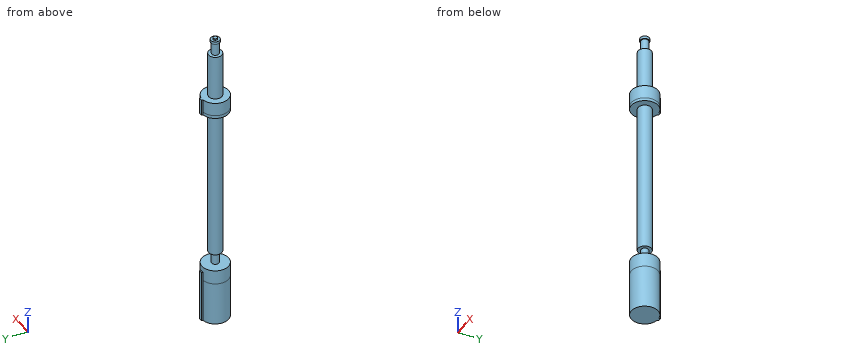
from build123d import *

# Parameters (mm, degrees)
CROQUIS1_R               = 4
SALIENTE_EXTRUIR1_DEPTH  = 135
CROQUIS2_R               = 5
SALIENTE_EXTRUIR2_DEPTH  = 3
SALIENTE_EXTRUIR3_DEPTH  = 1.8
CROQUIS4_R               = 7.5
SALIENTE_EXTRUIR4_DEPTH  = 120.9
CROQUIS5_R               = 15
SALIENTE_EXTRUIR5_DEPTH  = 15
CROQUIS7_W               = 4
CROQUIS7_H               = 3
SALIENTE_EXTRUIR6_DEPTH  = 15
SALIENTE_EXTRUIR7_DEPTH  = 3.4
CROQUIS9_R               = 15
SALIENTE_EXTRUIR8_DEPTH  = 6
CROQUIS10_R              = 15
SALIENTE_EXTRUIR9_DEPTH  = 10
SALIENTE_EXTRUIR10_DEPTH = 49


with BuildPart() as part:
    # Croquis1 → Saliente-Extruir1 (new, symmetric)
    with BuildSketch(Plane.XY):
        Circle(CROQUIS1_R)
    extrude(amount=SALIENTE_EXTRUIR1_DEPTH, both=True)

    # Croquis2 → Saliente-Extruir2 (add)
    with BuildSketch(Plane.XY.offset(135)):
        Circle(CROQUIS2_R)
    extrude(amount=SALIENTE_EXTRUIR2_DEPTH)

    # Croquis3 → Saliente-Extruir3 (add)
    with BuildSketch(Plane.XY.offset(138)):
        Polygon((0, 2.5), (-2.165063509, 1.25), (-2.165063509, -1.25), (0, -2.5), (2.165063509, -1.25), (2.165063509, 1.25), align=None)
    extrude(amount=SALIENTE_EXTRUIR3_DEPTH)

    # Croquis4 → Saliente-Extruir4 (add, symmetric)
    with BuildSketch(Plane.XY):
        Circle(CROQUIS4_R)
    extrude(amount=SALIENTE_EXTRUIR4_DEPTH, both=True)

    # Croquis5 → Saliente-Extruir5 (add)
    with BuildSketch(Plane(origin=(0, 0, 70), x_dir=(-1, 0, 0), z_dir=(0, 0, -1))):
        Circle(CROQUIS5_R)
    extrude(amount=SALIENTE_EXTRUIR5_DEPTH)

    # Croquis7 → Saliente-Extruir6 (add)
    with BuildSketch(Plane.XY.offset(70)):
        with Locations((0, 15)):
            Rectangle(CROQUIS7_W, CROQUIS7_H)
    extrude(amount=-SALIENTE_EXTRUIR6_DEPTH)

    # Croquis8 → Saliente-Extruir7 (add)
    with BuildSketch(Plane(origin=(0, 0, 55), x_dir=(-1, 0, 0), z_dir=(0, 0, -1))):
        with BuildLine():
            Line((2, 14.866068747), (2, 16.5))
            Line((2, 16.5), (-2, 16.5))
            Line((-2, 16.5), (-2, 14.866068747))
            ThreePointArc((-2, 14.866068747), (0, -15), (2, 14.866068747))
        make_face()
    extrude(amount=SALIENTE_EXTRUIR7_DEPTH)

    # Croquis9 → Saliente-Extruir8 (add)
    with BuildSketch(Plane(origin=(0, 0, -135), x_dir=(-1, 0, 0), z_dir=(0, 0, -1))):
        Circle(CROQUIS9_R)
    extrude(amount=SALIENTE_EXTRUIR8_DEPTH)

    # Croquis10 → Saliente-Extruir9 (add)
    with BuildSketch(Plane(origin=(0, 0, -141), x_dir=(-1, 0, 0), z_dir=(0, 0, -1))):
        with Locations(Location((0, 0, 0), (0, 0, 97.662255661))):
            Circle(CROQUIS10_R)
        with BuildLine():
            Line((-2, 16.5), (-2, 14.866068747))
            ThreePointArc((-2, 14.866068747), (0, 15), (2, 14.866068747))
            Line((2, 14.866068747), (2, 16.5))
            Line((2, 16.5), (-2, 16.5))
        make_face()
    extrude(amount=SALIENTE_EXTRUIR9_DEPTH)

    # Croquis11 → Saliente-Extruir10 (add)
    with BuildSketch(Plane(origin=(0, 0, -151), x_dir=(-1, 0, 0), z_dir=(0, 0, -1))):
        with BuildLine():
            Line((2, 14.866068747), (2, 16.5))
            Line((2, 16.5), (-2, 16.5))
            Line((-2, 16.5), (-2, 14.866068747))
            ThreePointArc((-2, 14.866068747), (0, -15), (2, 14.866068747))
        make_face()
    extrude(amount=SALIENTE_EXTRUIR10_DEPTH)


solid = part.part
The listing builds one solid part. Answer for the finished solid, in the listing's coordinates (mm). Round coordinates to 2 decimals unless told otherwise and drop trailing zeros. Write each loop counter-clockwise with the first axis right and the second up, starting at its lowest first coordinate (ties: lowest second). Pieces come first, ordered by that corner, then holes. Notation, with made-up numbers: M 74.5,-19 L 122.5,-19 A12 ccw 122.5,-13 Z; hole C -29.5,0.5 d9. An arc over 180 degrees is marked long. Write each question's results on one line, items separated by ' | '. Start each with the question number.
Item 1: Straight lines are drawn through the part: probe 1 along Z at (x, y) = (10.5, -7); probe 2 along X at (y, z) = (1, 103.5); probe 3 along Z at (x, y) = (-4, -4). For each, find the intervals that lie inside material, in ascending order.
Item 2: Given pin 1 Ø0.8 at (y, z) = (16, -183) entering from -X; pin 2 Ø2 at (y, z) = (0, 138.5) entering from -X; pin 3 Ø2 at (y, z) = (2, -77) entering from -X; pin 4 Ø3 at (y, z) = (-10, 94) entering from +X, each flat-ended and moving along its own axis, determine where each tip first touches the part or whether it passes through.
Item 3: Find section D-D on z = -161. Write down the section's boundary in (x, y).
Item 4: Find section A-A on y = -11.5. Write down the section's boundary in (x, z), and give its area (3 significant figures).
Item 5: Find section B-B on z = 74. Write down the section's boundary in (x, y).
Answer block:
1) probe 1: z = -200 to -135, 51.6 to 70 | probe 2: x = -7.43 to 7.43 | probe 3: z = -200 to -135, -120.9 to 120.9
2) pin 1: stops at x = -2 | pin 2: stops at x = -5 | pin 3: stops at x = -7.43 | pin 4: passes through
3) outline: M -2,14.87 A15 ccw long 2,14.87 L 2,16.5 L -2,16.5 Z
4) outline: M -9.63,-200 L 9.63,-200 L 9.63,-135 L -9.63,-135 Z; M -9.63,51.6 L 9.63,51.6 L 9.63,70 L -9.63,70 Z | area: 1,610 mm²
5) outline: C 0,0 d15
